```python
from build123d import *

# Parameters (mm, degrees)
F1_DEPTH = 53
F2_R     = 17.5
F3_DEPTH = 3
F4_R     = 5
F5_DEPTH = 25
F6_R     = 25
F7_DEPTH = 29


with BuildPart() as f1:
    # F0 (on Front) → F1 (new body, symmetric)
    with BuildSketch(Plane.XZ):
        Polygon((135, 57), (60, 257), (-60, 257), (-135, 57), (-135, -257), (135, -257), align=None)
    extrude(amount=F1_DEPTH, both=True)

    # F2 (on face) → F3 (join)
    with BuildSketch(Plane.XZ.offset(53)):
        with Locations((105, 43.7)):
            Circle(F2_R)
        with Locations((43.345646, 105.146778)):
            Circle(F2_R)
        with Locations((-43.7, 105)):
            Circle(F2_R)
        with Locations((-105.146778, 43.345646)):
            Circle(F2_R)
        with Locations((-105, -43.7)):
            Circle(F2_R)
        with Locations((-43.345646, -105.146778)):
            Circle(F2_R)
        with Locations((43.7, -105)):
            Circle(F2_R)
        with Locations((105.146778, -43.345646)):
            Circle(F2_R)
    extrude(amount=F3_DEPTH)

    # F4 (on face) → F5 (cut)
    with BuildSketch(Plane(origin=(0, 53, 0), x_dir=(-1, 0, 0), z_dir=(0, 1, 0))):
        Circle(F4_R)
        with Locations((0, 197)):
            Circle(F4_R)
        with Locations((0, -197)):
            Circle(F4_R)
    extrude(amount=-F5_DEPTH, mode=Mode.SUBTRACT)

    # F6 (on face) → F7 (join)
    with BuildSketch(Plane(origin=(0, 0, -257), x_dir=(1, 0, 0), z_dir=(0, 0, -1))):
        with Locations((106, 0)):
            Circle(F6_R)
        with Locations((-106, 0)):
            Circle(F6_R)
    extrude(amount=F7_DEPTH)


solid = f1.part
```
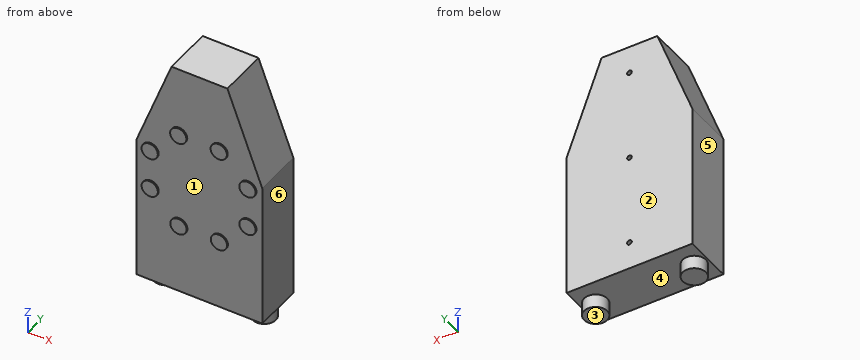
The listing builds one solid part. Answer for the finished solid, in the listing's coordinates (mm). Face numbers are marked on the shaded views. A direction names the side the tool comes from. Coordinates: 2 decimals unless noted, no trailing zeros. Loops run counter-clockwise (first coordinate to the right, second up) from the corner with the lowest first, then second, coordinate; pieces in that order, holes last. Notation, with made-up numbers: (-0.75, -27) -> (30.25, -27) arc R9 ccw to (30.25, -20) -> close; hole circle Ø7 at (49, -39). An arc over 180 degrees is marked (long way). Use one line per item in the form item = value. Start each with the question number.
Item 1: Flat-ended cylindrical pins translate along their axes: pin 1 Ø5 at (x, z) = (15.5, 15) entering from -Y; pin 2 Ø11.5 at (x, z) = (0, 0) entering from +Y; pin 3 Ø8 at (x, z) = (0, 197) entering from +Y. Find the tip coordinate at first contact, or state that the pin passes through.
Item 2: The part is cut by section D-D on z = 223. Determine the outline of the cut face in (x, y).
Item 3: The part is cut by section A-A on z = -197. Determine the outline of the cut face in (x, y).
Item 4: A tool of negligible diameter and unlimited length cuts with its end or side. For the marked faces 1 and 2, from which of +Z, -Z, +X, -X, +Y, -Y can it reach the whole face along a straight path? Write none if from no direction.
Item 5: The mould has two halves that part along X. Classify the marked faces 3, 4, 5 and 6: released by +X, released by -X, zero draft, split by the parting line, or undercut.
Item 6: The part is cut by section B-B on y = -45.5. Determine the outline of the cut face in (x, z).
Item 7: Consider L1, parallel to Z at x = 0, y = 42.5; L2, parallel to Y at x = -62, z = -83.5; L3, parallel to Z at x = 9.5, y = 30.5. Determine where each line is inside the solid, lowest interval first. Write a range as [from, to].
Item 8: The part is cut by section C-C on x = 35. Determine the outline of the cut face in (y, z).
Answer key:
q1.pin_1 = -53
q1.pin_2 = 53
q1.pin_3 = 28
q2.outline = (-72.75, -53) -> (72.75, -53) -> (72.75, 53) -> (-72.75, 53) -> close
q3.outline = (-135, -53) -> (135, -53) -> (135, 53) -> (5, 53) -> (5, 28) -> (-5, 28) -> (-5, 53) -> (-135, 53) -> close
q4.face_1 = -Y
q4.face_2 = +Z, -Z, +X, -X, +Y
q5.face_3 = zero draft
q5.face_4 = undercut
q5.face_5 = released by -X
q5.face_6 = released by +X
q6.outline = (-135, -257) -> (135, -257) -> (135, 57) -> (60, 257) -> (-60, 257) -> (-135, 57) -> close
q7.L1 = [-257, -202], [-192, -5], [5, 192], [202, 257]
q7.L2 = [-53, 53]
q7.L3 = [-257, 257]
q8.outline = (-56, -120.18) -> (-53, -120.18) -> (-53, -257) -> (53, -257) -> (53, 257) -> (-53, 257) -> (-53, 120.53) -> (-56, 120.53) -> (-56, 89.76) -> (-53, 89.76) -> (-53, -89.82) -> (-56, -89.82) -> close
